from build123d import *

# Parameters (mm, degrees)
SKETCH1_W           = 22
SKETCH1_H           = 13
BOSS_EXTRUDE1_DEPTH = 6
BOSS_EXTRUDE2_DEPTH = 2
BOSS_EXTRUDE3_DEPTH = 8
SKETCH4_R           = 1.525
SKETCH4_R_2         = 1.524
CUT_EXTRUDE1_DEPTH  = 36.566838488
SKETCH5_W           = 9
SKETCH5_H           = 4.088652256
CUT_EXTRUDE2_DEPTH  = 38.735924528
FILLET1_R           = 2
SKETCH6_W           = 12
SKETCH6_H           = 13.009000019
SKETCH6_W_2         = 15.838286437
CUT_EXTRUDE3_DEPTH  = 4
SKETCH7_W           = 2.5
SKETCH7_H           = 8
BOSS_EXTRUDE5_DEPTH = 3
FILLET3_R           = 2.5
FILLET4_R           = 2.5
SKETCH9_W           = 24
SKETCH9_H           = 8
CUT_EXTRUDE5_DEPTH  = 3
BOSS_EXTRUDE6_REACH = 35.526
SKETCH10_W          = 5
SKETCH10_H          = 2.5


with BuildPart() as part:
    # Sketch1 → Boss-Extrude1 (new body)
    with BuildSketch(Plane(origin=(0, 0, 0), x_dir=(1, 0, 0), z_dir=(0, 1, 0))):
        with BuildLine():
            Line((-1, -3), (23, -3))
            Line((23, -3), (25, -3))
            Line((25, -3), (25, -1))
            Line((25, -1), (25, 14))
            Line((25, 14), (25, 16))
            Line((25, 16), (23, 16))
            Line((23, 16), (-1, 16))
            ThreePointArc((-1, 16), (-2.414213562, 15.414213562), (-3, 14))
            Line((-3, 14), (-3, -1))
            ThreePointArc((-3, -1), (-2.414213562, -2.414213562), (-1, -3))
        make_face()
        with Locations((11, 6.5)):
            Rectangle(SKETCH1_W, SKETCH1_H, mode=Mode.SUBTRACT)
    extrude(amount=BOSS_EXTRUDE1_DEPTH)

    # Sketch2 → Boss-Extrude2 (add)
    with BuildSketch(Plane(origin=(0, 6, 0), x_dir=(1, 0, 0), z_dir=(0, 1, 0))):
        with BuildLine():
            Line((25, 14), (25, -1))
            Line((25, -1), (25, -3))
            Line((25, -3), (23, -3))
            Line((23, -3), (-1, -3))
            ThreePointArc((-1, -3), (-2.414213562, -2.414213562), (-3, -1))
            Line((-3, -1), (-3, 14))
            ThreePointArc((-3, 14), (-2.414213562, 15.414213562), (-1, 16))
            Line((-1, 16), (23, 16))
            Line((23, 16), (25, 16))
            Line((25, 16), (25, 14))
        make_face()
    extrude(amount=BOSS_EXTRUDE2_DEPTH)

    # Sketch3 → Boss-Extrude3 (add)
    with BuildSketch(Plane.XZ):
        with BuildLine():
            Line((5, 3), (17, 3))
            Line((17, 3), (17, 5.5))
            ThreePointArc((17, 5.5), (15.389087297, 9.389087297), (11.5, 11))
            Line((11.5, 11), (10.5, 11))
            ThreePointArc((10.5, 11), (6.610912703, 9.389087297), (5, 5.5))
            Line((5, 5.5), (5, 3))
        make_face()
        with BuildLine():
            Line((17, -16), (5, -16))
            Line((5, -16), (5, -18.5))
            ThreePointArc((5, -18.5), (6.610912703, -22.389087297), (10.5, -24))
            Line((10.5, -24), (11.5, -24))
            ThreePointArc((11.5, -24), (15.389087297, -22.389087297), (17, -18.5))
            Line((17, -18.5), (17, -16))
        make_face()
    extrude(amount=-BOSS_EXTRUDE3_DEPTH)

    # Sketch4 → Cut-Extrude1 (cut, through all)
    with BuildSketch(Plane(origin=(0, 0, 0), x_dir=(-1, 0, 0), z_dir=(0, -1, 0))):
        with Locations(Location((-11, 20, 0), (0, 0, 90))):
            Circle(SKETCH4_R)
        with Locations(Location((-11, -7, 0), (0, 0, 90))):
            Circle(SKETCH4_R_2)
    extrude(amount=-CUT_EXTRUDE1_DEPTH, mode=Mode.SUBTRACT)

    # Sketch5 → Cut-Extrude2 (cut, through all)
    with BuildSketch(Plane(origin=(25, 0, 0), x_dir=(0, 0, -1), z_dir=(1, 0, 0))):
        with Locations((6.5, 2.044326128)):
            Rectangle(SKETCH5_W, SKETCH5_H)
    extrude(amount=-CUT_EXTRUDE2_DEPTH, mode=Mode.SUBTRACT)

    # Fillet1
    fillet1_edges = [part.edges().sort_by_distance(p)[0] for p in [
        (-1.5, 4.088652256, -11),
        (-1.5, 4.088652256, -2),
        (23.5, 4.088652256, -11),
        (23.5, 4.088652256, -2),
    ]]
    fillet(fillet1_edges, radius=FILLET1_R)

    # Sketch6 → Cut-Extrude3 (cut)
    with BuildSketch(Plane(origin=(0, 8, 0), x_dir=(1, 0, 0), z_dir=(0, 1, 0))):
        with Locations((11, 22.504500009)):
            Rectangle(SKETCH6_W, SKETCH6_H)
        with Locations((11.149066226, -9.50450001)):
            Rectangle(SKETCH6_W_2, SKETCH6_H)
    extrude(amount=-CUT_EXTRUDE3_DEPTH, mode=Mode.SUBTRACT)

    # Sketch7 → Boss-Extrude5 (add)
    with BuildSketch(Plane(origin=(25, 0, 0), x_dir=(0, 0, -1), z_dir=(1, 0, 0))):
        with Locations((17.25, 4)):
            Rectangle(SKETCH7_W, SKETCH7_H)
        with Locations((-4.25, 4)):
            Rectangle(SKETCH7_W, SKETCH7_H)
    extrude(amount=-BOSS_EXTRUDE5_DEPTH)

    # Fillet3
    fillet3_edges = [part.edges().sort_by_distance(p)[0] for p in [
        (22, 4, -16),
    ]]
    fillet(fillet3_edges, radius=FILLET3_R - 0.0001)  # a hair under: the kernel refuses the full size

    # Fillet4
    fillet4_edges = [part.edges().sort_by_distance(p)[0] for p in [
        (22, 4, 3),
    ]]
    fillet(fillet4_edges, radius=FILLET4_R - 0.0001)  # a hair under: the kernel refuses the full size

    # Sketch9 → Cut-Extrude5 (cut)
    with BuildSketch(Plane(origin=(25, 0, 0), x_dir=(0, 0, -1), z_dir=(1, 0, 0))):
        with Locations((6.5, 4)):
            Rectangle(SKETCH9_W, SKETCH9_H)
    extrude(amount=-CUT_EXTRUDE5_DEPTH, mode=Mode.SUBTRACT)

    # Boss-Extrude6: up to this face of the body (flat: up to its plane)
    boss_extrude6_end = Plane(part.part.faces().sort_by_distance((9.97036164, 0, 3.836684907))[0])
    # Sketch10 → Boss-Extrude6 (add, up to the picked face)
    with BuildSketch(Plane(origin=(0, 8, 0), x_dir=(1, 0, 0), z_dir=(0, 1, 0)), mode=Mode.PRIVATE) as boss_extrude6_sk1:
        with Locations((19.5, 17.25)):
            Rectangle(SKETCH10_W, SKETCH10_H)
    boss_extrude6_tool1 = split(extrude(boss_extrude6_sk1.sketch, amount=-BOSS_EXTRUDE6_REACH, mode=Mode.PRIVATE), bisect_by=boss_extrude6_end, keep=Keep.BOTH, mode=Mode.PRIVATE)
    # Sketch10 → Boss-Extrude6 (add, up to the picked face)
    with BuildSketch(Plane(origin=(0, 8, 0), x_dir=(1, 0, 0), z_dir=(0, 1, 0)), mode=Mode.PRIVATE) as boss_extrude6_sk2:
        with Locations((19.5, -4.25)):
            Rectangle(SKETCH10_W, SKETCH10_H)
    boss_extrude6_tool2 = split(extrude(boss_extrude6_sk2.sketch, amount=-BOSS_EXTRUDE6_REACH, mode=Mode.PRIVATE), bisect_by=boss_extrude6_end, keep=Keep.BOTH, mode=Mode.PRIVATE)
    add(boss_extrude6_tool1.solids().sort_by(Axis((19.5, 8, -17.25), (0, -1, 0)))[0])
    add(boss_extrude6_tool2.solids().sort_by(Axis((19.5, 8, 4.25), (0, -1, 0)))[0])


solid = part.part
Geometry: final body of the model. Coordinates: model frame, mm. A direction names the side the tool comes from. Give positions to 0.01 mm unless a question says otherwise; leave off trailing zeros. Order: outer loops, then holes, each group sorted by start corner. A loop starts at its lowest first (then second) coordinate and runs counter-clockwise, first axis right, second up. Notation, with made-up numbers: (-18.5, 7.5) - (4.5, 7.5) arc R14 cw to (4.5, 19.5) - close; hole circle Ø1 at (7.5, 26). An arc over 180 degrees is marked (long way). Use CSV: the item, a comma, the result in double quotes.
1. Section query B-B (y = 3). Output: boundary loops of the cut face in (x, z) (3 decimals).
Answers below:
outline,"(-3, -14) arc R2 ccw to (-1, -16) - (5, -16) - (5, -18.5) arc R5.5 ccw to (10.5, -24) - (11.5, -24) arc R5.5 ccw to (17, -18.5) - (22, -18.5) - (22, -13) - (0, -13) - (0, -10.78) - (-3, -10.78) - close; (-3, -2.22) - (0, -2.22) - (0, 0) - (22, 0) - (22, 5.5) - (17, 5.5) arc R5.5 ccw to (11.5, 11) - (10.5, 11) arc R5.5 ccw to (5, 5.5) - (5, 3) - (-1, 3) arc R2 ccw to (-3, 1) - close; hole circle Ø3.05 at (11, -20); hole circle Ø3.048 at (11, 7)"
2. Mould query, pull axis Z, two halves, no side actions, for faces 4 (the face through (11, 2, 11)), 5 (the face through (6.57, 1.97, -22.35)), 6 (the face through (5, 2, 4)), 7 (the face through (-1, 4.089, -6)). Classes: +Z half, -Z half, draft (parallel to the pull), parting line (faces both ways), or undercut.
Answers below:
face 4,"+Z half"
face 5,"-Z half"
face 6,"draft"
face 7,"undercut"
3. Section query D-D (x = 3.25). Output: boundary loops of the cut face in (y, z), plus the area to 3 significant figures.
Answers below:
outline,"(0, -16) - (8, -16) - (8, 3) - (0, 3) - (0, 0) - (6, 0) - (6, -13) - (0, -13) - close"
area,"74.0 mm2"
4. Material intervals for line 1 along Z through (x, y) = (21.25, 3); line 2 along Z through (x, y) = (14.5, 5.5); line 3 along Z through (x, y) = (16.25, 6.5), sorted ascending. Write a range as from..to.
Answers below:
line 1,"-18.5..-13, 0..5.5"
line 2,"-16..-13, 0..3"
line 3,"-16..3"
5. Access query for faces 1 (the face through (11, 6, -7)), 2 (the face through (11, 4, -18)), 3 (the face through (9.58, 4, 6.06)). Directions: +Z, -Z, +X, -X, +Y, -Y. A direction counts if a zero-diameter tool reaches every point of the face in a straight line with its end or side. Return the directions, or none.
Answers below:
face 1,"+X, -Y"
face 2,"-Z, -X, +Y"
face 3,"+Z, -X, +Y"
6. Section query A-A (x = 11). Output: boundary loops of the cut face in (y, z) (3 decimals), plus the area to 3 significant figures.
Answers below:
outline,"(0, -24) - (4, -24) - (4, -21.525) - (0, -21.525) - close; (0, -18.475) - (4, -18.475) - (4, -16) - (8, -16) - (8, 3) - (4, 3) - (4, 5.476) - (0, 5.476) - (0, 0) - (6, 0) - (6, -13) - (0, -13) - close; (0, 8.524) - (4, 8.524) - (4, 11) - (0, 11) - close"
area,"114 mm2"
7. Contact query for flat-ended pins moving along their axis: pin 1 (3.5 mm diameter, centred on x = -1, z = -6, fed in from -Y); pin 2 (1 mm diameter, centred on x = 17, y = 5.5, fed in from -Z); pin 3 (10.5 mm diameter, centred on x = 14.5, z = -6, fed in from -Y). Output: stop coordinate, or through.
Answers below:
pin 1,"y = 4.09"
pin 2,"z = -18.5"
pin 3,"y = 6"
8. Section query C-C (z = -20). Output: boundary loops of the cut face in (x, y) (1 decimal), plus the area to 3 significant figures.
Answers below:
outline,"(5.2, 0) - (9.5, 0) - (9.5, 4) - (5.2, 4) - close; (12.5, 0) - (16.8, 0) - (16.8, 4) - (12.5, 4) - close"
area,"34.1 mm2"
